from build123d import *

# Parameters (mm, degrees)
BOSS_EXTRUDE1_DEPTH     = 37.5
CUT_EXTRUDE1_DEPTH      = 46.067643604
CUT_EXTRUDE1_DEPTH_BACK = 46.067643604
SKETCH2_W               = 8
SKETCH2_H               = 16
CUT_EXTRUDE2_DEPTH      = 46.067643604
CUT_EXTRUDE2_DEPTH_BACK = 46.067643604
SKETCH3_W               = 8
SKETCH3_H               = 13.5
SKETCH4_R               = 3
CUT_EXTRUDE3_DEPTH      = 46.067643604
LPATTERN1_COUNT         = 2
LPATTERN1_PITCH         = 28
MIRROR1_COPY_1_SKETCH_R = 3
MIRROR1_COPY_1_DEPTH    = 46.067643604
MIRROR1_COPY_2_SKETCH_R = 3
MIRROR1_COPY_2_DEPTH    = 46.067643604
CHAMFER1_SIZE           = 1.2


with BuildPart() as part:
    # Sketch1 → Boss-Extrude1 (new, symmetric)
    with BuildSketch(Plane.XY):
        with BuildLine():
            Line((1.865475811, 3.15), (24.45, 3.15))
            Line((24.45, 3.15), (24.45, 1.65))
            Line((24.45, 1.65), (1.509966887, 1.65))
            ThreePointArc((1.509966887, 1.65), (1.253893127, 1.683342755), (1.014895777, 1.781147541))
            ThreePointArc((1.014895777, 1.781147541), (-1.507477704, -1.389248347), (1.857930963, 0.866367437))
            Line((1.857930963, 0.866367437), (3.217392644, 1.500294829))
            ThreePointArc((3.217392644, 1.500294829), (-2.492742617, -2.527594557), (1.455481127, 3.237912088))
            ThreePointArc((1.455481127, 3.237912088), (1.655818843, 3.172224997), (1.865475811, 3.15))
        make_face()
    extrude(amount=BOSS_EXTRUDE1_DEPTH, both=True)

    # Sketch2 → Cut-Extrude1 (cut, two sides: drawn at the far end of the back side and taken through both)
    with BuildSketch(Plane.XZ.offset(-1.65).offset(-CUT_EXTRUDE1_DEPTH_BACK)):
        with Locations((0.45, 0)):
            Rectangle(SKETCH2_W, SKETCH2_H)
    extrude(amount=CUT_EXTRUDE1_DEPTH + CUT_EXTRUDE1_DEPTH_BACK, mode=Mode.SUBTRACT)

    # Sketch3 → Cut-Extrude2 (cut, two sides: drawn at the far end of the back side and taken through both)
    with BuildSketch(Plane.XZ.offset(-1.65).offset(-CUT_EXTRUDE2_DEPTH_BACK)):
        with Locations((0.45, 30.75)):
            Rectangle(SKETCH3_W, SKETCH3_H)
        with Locations((0.45, -30.75)):
            Rectangle(SKETCH3_W, SKETCH3_H)
    extrude(amount=CUT_EXTRUDE2_DEPTH + CUT_EXTRUDE2_DEPTH_BACK, mode=Mode.SUBTRACT)

    # Sketch4 → Cut-Extrude3 (cut, through all)
    with BuildSketch(Plane.XZ.offset(-1.65)):
        with Locations(Location((15.45, 0, 0), (0, 0, 270))):
            Circle(SKETCH4_R)
    cut_extrude3 = extrude(amount=-CUT_EXTRUDE3_DEPTH, mode=Mode.SUBTRACT)

    # LPattern1: Cut-Extrude3 ×2
    with Locations(*[(0, 0, -i * LPATTERN1_PITCH) for i in range(1, LPATTERN1_COUNT)]):
        add(cut_extrude3, mode=Mode.SUBTRACT)

    # Mirror1 copy 1 sketch → Mirror1 copy 1 (cut, through all)
    with BuildSketch(Plane(origin=(0, 1.65, 28), x_dir=(1, 0, 0), z_dir=(0, -1, 0))):
        with Locations((15.45, 0)):
            Circle(MIRROR1_COPY_1_SKETCH_R)
    extrude(amount=-MIRROR1_COPY_1_DEPTH, mode=Mode.SUBTRACT)

    # Mirror1 copy 2 sketch → Mirror1 copy 2 (cut, through all)
    with BuildSketch(Plane.XZ.offset(-1.65)):
        with Locations((15.45, 0)):
            Circle(MIRROR1_COPY_2_SKETCH_R)
    extrude(amount=-MIRROR1_COPY_2_DEPTH, mode=Mode.SUBTRACT)

    # Chamfer1
    chamfer1_edges = [part.edges().sort_by_distance(p)[0] for p in [
        (15.45, 1.65, 3),
        (15.45, 1.65, -25),
        (12.45, 1.65, 28),
    ]]
    chamfer(chamfer1_edges, length=CHAMFER1_SIZE)


solid = part.part
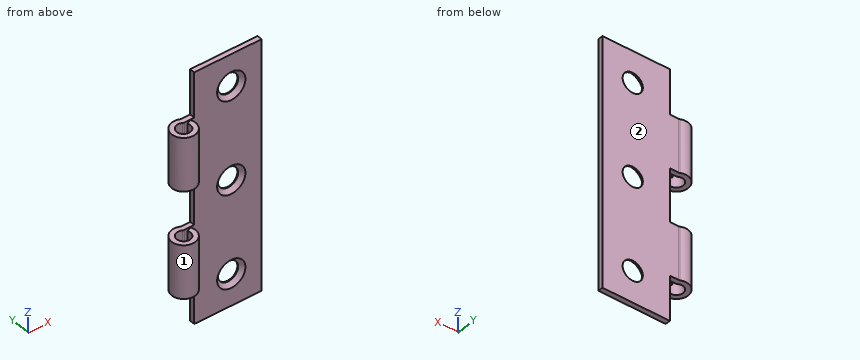
The model under review builds one solid part; all positions refer to its coordinate system, in mm. Face numbers are marked on the shaded views. A direction names the side the tool comes from. Round coordinates to 2 decimals unless told otherwise and drop trailing zeros. Loops run counter-clockwise (first coordinate to the right, second up) from the corner with the lowest first, then second, coordinate; pieces in that order, holes last. Notation, with made-up numbers: (52, 43.25) -> (93, 43.25) arc R24 ccw to (93, 61.25) -> close; hole circle Ø5 at (42, 27.25). An arc over 180 degrees is marked (long way). Return JSON: item names as keys, results as strings.
(1) Add section C-C on z = -11.5. Write out the cut boundary in (x, y).
Solved:
{"outline": "(1.01, 1.78) arc R1 ccw to (1.51, 1.65) -> (24.45, 1.65) -> (24.45, 3.15) -> (1.87, 3.15) arc R1 cw to (1.46, 3.24) arc R3.55 ccw (long way) to (3.22, 1.5) -> (1.86, 0.87) arc R2.05 cw (long way) to start"}
(2) Add section D-D on y = -1.25. Write out the cut boundary in (x, z).
Solved:
{"outline": "(-3.32, -24) -> (-1.62, -24) -> (-1.62, -8) -> (-3.32, -8) -> close; (-3.32, 8) -> (-1.62, 8) -> (-1.62, 24) -> (-3.32, 24) -> close; (1.62, -24) -> (3.32, -24) -> (3.32, -8) -> (1.62, -8) -> close; (1.62, 8) -> (3.32, 8) -> (3.32, 24) -> (1.62, 24) -> close"}
(3) For pin 1 (3 mm diameter, centred on x = 5.5, z = -10, fed in from -Y); pin 2 (3.5 mm diameter, centred on x = 0, y = 1.5, fed in from +Z); pin 3 (8 mm diameter, centred on x = 4.5, z = -19.5, fed in from -Y); pin 4 (5 mm diameter, centred on x = 15.45, z = 0, fed in from +Y), all flat-tipped, find the tip position at first contact; note any pin that passes through.
Solved:
{"pin 1": "y = 1.65", "pin 2": "z = 24", "pin 3": "y = -3.51", "pin 4": "through"}
(4) For line 1 (X direction, y = 3, z = 0); line 2 (X direction, y = 0, z = -17); line 3 (Z direction, x = 0, y = -2.5), list the stretches that pass through material, from the lowest coordinate up.
Solved:
{"line 1": "4.45 to 12.45, 18.45 to 24.45", "line 2": "-3.55 to -2.05, 2.05 to 3.55", "line 3": "-24 to -8, 8 to 24"}
(5) Add section A-A on x = 0. Write out the cut boundary in (y, z).
Solved:
{"outline": "(-3.55, -24) -> (-2.05, -24) -> (-2.05, -8) -> (-3.55, -8) -> close; (-3.55, 8) -> (-2.05, 8) -> (-2.05, 24) -> (-3.55, 24) -> close; (2.05, -24) -> (3.55, -24) -> (3.55, -8) -> (2.05, -8) -> close; (2.05, 8) -> (3.55, 8) -> (3.55, 24) -> (2.05, 24) -> close"}
(6) Add section B-B on z = 28. Write out the cut boundary in (x, y).
Solved:
{"outline": "(4.45, 1.65) -> (11.25, 1.65) -> (12.45, 2.85) -> (12.45, 3.15) -> (4.45, 3.15) -> close; (18.45, 2.85) -> (19.65, 1.65) -> (24.45, 1.65) -> (24.45, 3.15) -> (18.45, 3.15) -> close"}
(7) For the marked faces 1 and 2, list the 3-axis set-ups (+Z, -Z, +X, -X, +Y, -Y) from which the entire face can be reached by the end or side of a thin tool; tool diameter is ignored.
Solved:
{"face 1": "+Z, -Z", "face 2": "+Z, -Z, +X, +Y"}
